```python
from build123d import *

# Parameters (mm, degrees)
F1_DEPTH = 0.794
F2_R     = 1.6195
F3_DEPTH = 25


with BuildPart() as f1:
    # F0 (on Top) → F1 (new body, symmetric)
    with BuildSketch(Plane.XY):
        Polygon((32.02, 26.67), (-32.02, 26.67), (-32.02, 0), (-32.02, -26.67), (32.02, -26.67), (32.02, -24.003), (34.56, -21.463), (34.56, 11.557), (32.02, 14.097), align=None)
    extrude(amount=F1_DEPTH, both=True)

    # F2 (on face) → F3 (cut)
    with BuildSketch(Plane.XY.offset(0.794)):
        with Locations((-16.863, 23.959)):
            Circle(F2_R)
        with Locations((-18.006, -23.959)):
            Circle(F2_R)
        with Locations((31.925, 3.538941)):
            Circle(F2_R)
        with Locations((31.925, -19.209)):
            Circle(F2_R)
    extrude(amount=-F3_DEPTH, mode=Mode.SUBTRACT)


solid = f1.part
```
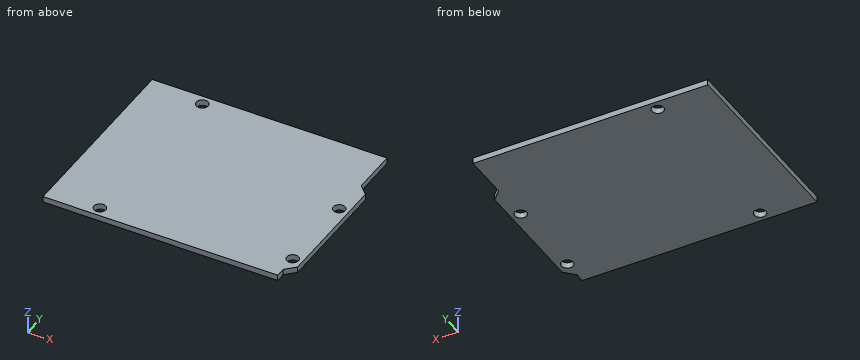
Here's how the part is built. I have some questions about the finished solid (model axes, mm). Round coordinates to 2 decimals unless told otherwise and drop trailing zeros. Order: outer loops, then holes, each group sorted by start corner. A loop starts at its lowest first (then second) coordinate and runs counter-clockwise, first axis right, second up. Notation, with made-up numbers: (-40, 56.25) -> (15, 56.25) arc R7 ccw to (15, 66.25) -> close; hole circle Ø9 at (-26, 44.5). An arc over 180 degrees is marked (long way). Use a Markdown table: item, result. Add a question column.
(1) Suppose I cut it at B-B, the plane z = 0.3. Please give me the cut outline in (x, y) (1 decimal).
(2) Suppose I cut it at A-A, the plane y = -20. Please give me the cut outline in (x, z), and give its area (3 significant figures).
(3) I need wall thicknesses on line 1 along X through (y, z) = (-24, -0.1); line 2 along X through (y, z) = (-19, -0.35); line 3 along Y through (x, z) = (-18, -0.15). Which ranges of each line are inside material? Lowest first, please.
Verdict:
| question | item | result |
|---|---|---|
| 1 | outline | (-32, -26.7) -> (32, -26.7) -> (32, -24) -> (34.6, -21.5) -> (34.6, 11.6) -> (32, 14.1) -> (32, 26.7) -> (-32, 26.7) -> close; hole circle Ø3.2 at (-18, -24); hole circle Ø3.2 at (-16.9, 24); hole circle Ø3.2 at (31.9, -19.2); hole circle Ø3.2 at (31.9, 3.5) |
| 2 | outline | (-32.02, -0.79) -> (30.51, -0.79) -> (30.51, 0.79) -> (-32.02, 0.79) -> close; (33.34, -0.79) -> (34.56, -0.79) -> (34.56, 0.79) -> (33.34, 0.79) -> close |
| 2 | area | 101 mm2 |
| 3 | line 1 | -32.02 to -19.62, -16.39 to 32.02 |
| 3 | line 2 | -32.02 to 30.32, 33.53 to 34.56 |
| 3 | line 3 | -26.67 to -25.58, -22.34 to 22.81, 25.11 to 26.67 |
